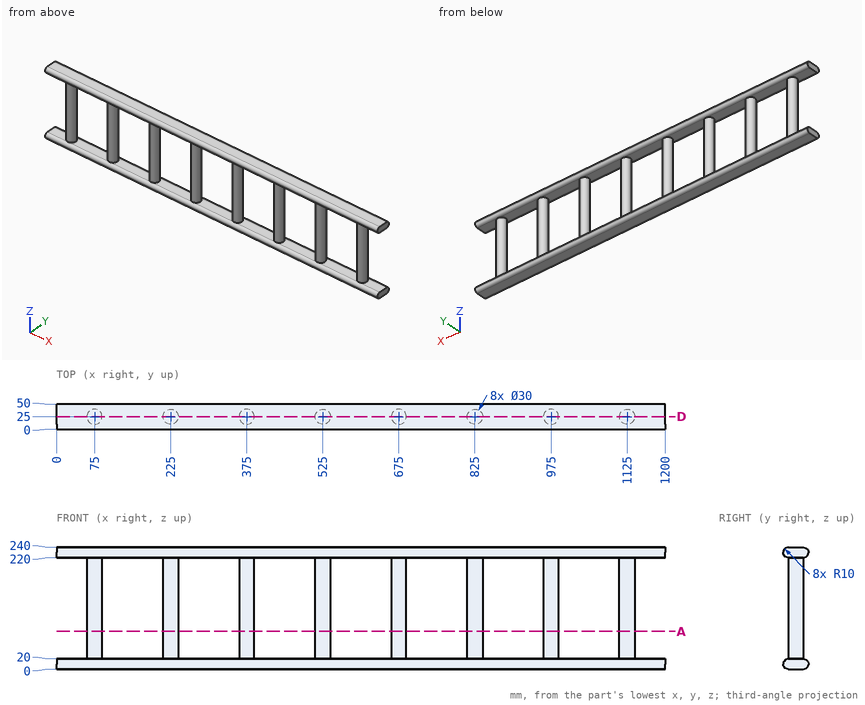
Geometry: see drawing. Coordinates: mm, zero at the bounding-box minimum. Coordinates: 2 decimals unless noted, no trailing zeros. Loops run counter-clockwise (first coordinate to the right, second up) from the corner with the lowest first, then second, coordinate; pieces in that order, holes last.
Q1. Cut plane D-D (y = 25). Give the number of separate pieces and of enclosed holes in the cut face, then the cut area to 3 significant figures.
Q2. Contact query for flat-ended pins moving along their axis: pin 1 (1 mm diameter, centred on x = 512, z = 156.5, fed in from +Y); pin 2 (8 mm diameter, centred on y = 8.5, z = 201.5, fed in from -X); pin 3 (1.5 mm diameter, centred on x = 185.5, y = 43.5, fed in from +Z); pin 4 (1.5 mm diameter, centred on x = 960, y = 21, fed in from -Z). Output: stop coordinate, or through.
Q3. Cut plane A-A (z = 74.5). Output: boundary loops of the cut face in (x, y).
Q4. Material intervals for line 1 (Z direction, x = 980.5, y = 41); line 2 (Z direction, x = 125.5, y = 26), sorted ascending.
Working result:
1. separate pieces: 1
1. enclosed holes: 7
1. area: 96,000 mm2
2. pin 1: stops at y = 33.29
2. pin 2: stops at x = 66.71
2. pin 3: stops at z = 239.61
2. pin 4: stops at z = 0
3. outline: circle Ø30 at (75, 25); circle Ø30 at (225, 25); circle Ø30 at (375, 25); circle Ø30 at (525, 25); circle Ø30 at (675, 25); circle Ø30 at (825, 25); circle Ø30 at (975, 25); circle Ø30 at (1125, 25)
4. line 1: z = 0.05 to 19.95, 220.05 to 239.95
4. line 2: z = 0 to 20, 220 to 240
